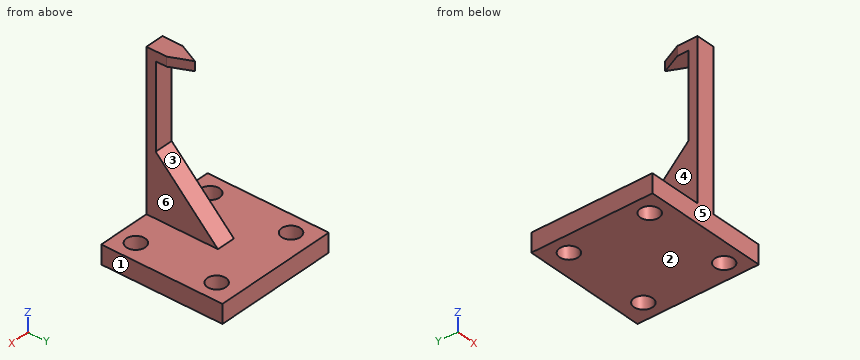
from build123d import *

# Parameters (mm, degrees)
BOSS_EXTRUDE1_DEPTH = 1.5
SKETCH2_W           = 3
SKETCH2_H           = 1.5
BOSS_EXTRUDE2_DEPTH = 5
SKETCH3_W           = 20
SKETCH3_H           = 3
BOSS_EXTRUDE3_DEPTH = 18
CUT_EXTRUDE1_DEPTH  = 10
SKETCH5_R           = 1.5
CUT_EXTRUDE4_DEPTH  = 10
BOSS_EXTRUDE4_DEPTH = 3


with BuildPart() as part:
    # Sketch1 → Boss-Extrude1 (new body)
    with BuildSketch(Plane(origin=(0, 0, 0), x_dir=(1, 0, 0), z_dir=(0, 1, 0))):
        Polygon((3, 25), (11.5, 25), (11.5, 28), (-8.5, 28), (-8.5, 25), (0, 25), (0, 0), (3, 0), align=None)
    extrude(amount=BOSS_EXTRUDE1_DEPTH)

    # Sketch2 → Boss-Extrude2 (add)
    with BuildSketch(Plane(origin=(0, 1.5, 0), x_dir=(1, 0, 0), z_dir=(0, 1, 0))):
        with Locations((1.5, 0.75)):
            Rectangle(SKETCH2_W, SKETCH2_H)
    extrude(amount=BOSS_EXTRUDE2_DEPTH)

    # Sketch3 → Boss-Extrude3 (add)
    with BuildSketch(Plane(origin=(0, 1.5, 0), x_dir=(1, 0, 0), z_dir=(0, 1, 0))):
        with Locations((1.5, 26.5)):
            Rectangle(SKETCH3_W, SKETCH3_H)
    extrude(amount=BOSS_EXTRUDE3_DEPTH)

    # Sketch4 → Cut-Extrude1 (cut)
    with BuildSketch(Plane.XY):
        Polygon((1.5, 6.5), (0, 3.25), (-1.660876249, 3.25), (-2.026223081, 8.127487576), (5.302958893, 8.676477884), (5.709427688, 3.25), (3, 3.25), align=None)
    extrude(amount=-CUT_EXTRUDE1_DEPTH, mode=Mode.SUBTRACT)

    # Sketch5 → Cut-Extrude4 (cut)
    with BuildSketch(Plane.XY.offset(-25)):
        with Locations((-5.5, 3)):
            Circle(SKETCH5_R)
        with Locations((8.5, 3)):
            Circle(SKETCH5_R)
        with Locations((8.5, 16)):
            Circle(SKETCH5_R)
        with Locations((-5.5, 16)):
            Circle(SKETCH5_R)
    extrude(amount=-CUT_EXTRUDE4_DEPTH, mode=Mode.SUBTRACT)

    # Sketch6 → Boss-Extrude4 (add)
    with BuildSketch(Plane.ZY):
        Polygon((-25, 1.5), (-25, 11.5), (-15, 1.5), align=None)
    extrude(amount=-BOSS_EXTRUDE4_DEPTH)


solid = part.part
Design review of the part built by this model. Coordinates are the model's own, in mm. Face numbers are marked on the shaded views. A direction names the side the tool comes from. Give positions to 0.01 mm unless a question says otherwise; leave off trailing zeros. Write each loop counter-clockwise with the first axis right and the second up, starting at its lowest first coordinate (ties: lowest second). Pieces come first, ordered by that corner, then holes. Notation, with made-up numbers: M -16.5,-26.5 L -12.5,-26.5 A30 ccw -12.5,3.5 Z; hole C -5.5,-8.5 d9. An arc over 180 degrees is marked long. Return JSON: item names as keys, results as strings. Group by question number.
Item 1: Take a section at C-C (z = -6). Give the boundary of the cut face in (x, y), plus the area to 3 significant figures.
Item 2: Clearance check with flat-ended pins moving along their axes: pin 1 Ø6 at (y, z) = (4, -6.5) entering from +X; pin 2 Ø10 at (y, z) = (2.5, -18) entering from -X; pin 3 Ø2.5 at (x, z) = (1.5, -6) entering from +Y. State where each tip first meets the part, or that it passes through.
Item 3: The part is to be moulded in two halves that separate along Z. For the marked faces 1, 2 and 3, say which applies: pulls with the +Z half, pulls with the -Z half, needs draft (parallel to the pull), parting line crosses it, or undercut.
Item 4: Tool access review of the marked faces 4, 5 and 6: name each direction out of +Z, -Z, +X, -X, +Y, -Y from which nothing blocks a thin tool from reaching the whole face with its end or side.
Item 5: Take a section at D-D (x = 4). Give the boundary of the cut face in (y, z), plus the area to 3 significant figures.
Item 6: Wall thickness on line 1 along Y through (x, z) = (8.5, -26.7); line 2 along Z through (x, y) = (3, 16.75); line 3 along Z through (x, y) = (2.75, 10.25): over which ranges is each line inside the solid? List them lowest first.
Item 7: Take a section at A-A (y = 16). Give the boundary of the cut face in (x, z).
Item 8: Take a section at B-B (x = -5.5). Give the boundary of the cut face in (y, z), plus the area to 3 significant figures.
Return value:
{
 "1": {"outline": "M 0,0 L 3,0 L 3,1.5 L 0,1.5 Z", "area": "4.50 mm2"},
 "2": {"pin 1": "stops at x = 3", "pin 2": "stops at x = 0", "pin 3": "stops at y = 1.5"},
 "3": {"face 1": "needs draft", "face 2": "pulls with the -Z half", "face 3": "undercut"},
 "4": {"face 4": "+Z, -X, +Y, -Y", "face 5": "+Z, -Z, +X, -X, -Y", "face 6": "+Z, +X, +Y, -Y"},
 "5": {"outline": "M 0,-28 L 19.5,-28 L 19.5,-25 L 0,-25 Z", "area": "58.5 mm2"},
 "6": {"line 1": "y = 0 to 1.5, 4.5 to 14.5, 17.5 to 19.5", "line 2": "z = -28 to -25", "line 3": "z = -28 to -23.75"},
 "7": {"outline": "M -8.5,-28 L -7,-28 L -7,-25 L -8.5,-25 Z; M -4,-28 L 7,-28 L 7,-25 L -4,-25 Z; M 10,-28 L 11.5,-28 L 11.5,-25 L 10,-25 Z"},
 "8": {"outline": "M 0,-28 L 1.5,-28 L 1.5,-25 L 0,-25 Z; M 4.5,-28 L 14.5,-28 L 14.5,-25 L 4.5,-25 Z; M 17.5,-28 L 19.5,-28 L 19.5,-25 L 17.5,-25 Z", "area": "40.5 mm2"}
}
